Autodesk Inventor part; units mm, degrees
ref_plane "YZ Plane" through (0, 0, 0) normal (1, 0, 0) x (0, 1, 0)
ref_plane "XZ Plane" through (0, 0, 0) normal (0, 1, 0) x (-1, 0, 0)
ref_plane "XY Plane" through (0, 0, 0) normal (0, 0, 1) x (1, 0, 0)
sketch "Sketch1" plane through (0, 0, 0) normal (0, 0, 1) x (1, 0, 0)
  circle A0 centre (0, 0) radius 6.858
  dimension "d0" = 13.716
extrude "Extrusion1" add sketch "Sketch1" along normal blind 13.716
hole "Hole1" at (0, 0, 13.716) direction (0, 0, -1) diameter 12.192 depth 3.048
hole "Hole2" at (0, 0, 10.668) direction (0, 0, -1) diameter 11.43 depth 9.144
sketch "Sketch2" plane through (0, 0, 0) normal (1, 0, 0) x (0, 1, 0)
  line L0 (0, 0) -> (0, 6.35)
  circle A0 centre (0, 6.35) radius 1.7399
  dimension "d21" = 6.35
  dimension "d22" = 3.4798
extrude "Extrusion2" cut sketch "Sketch2" along normal through all both and the other way through all
sketch "Sketch3" plane through (0, 0, 0) normal (0, 0, -1) x (-1, 0, 0)
  line L0 (0, 0) -> (4.8942, 4.8942)
  line L1 (0, 0) -> (0, 6.9215) construction
sketch "Sketch4" plane through (0, 0, 0) normal (0, 1, 0) x (-1, 0, 0)
  point P0 (0, 0)
ref_plane "Work Plane1" through (-4.8942, 4.8942, 0) normal (-0.7071, 0.7071, 0) x (-0.7071, -0.7071, 0)
sketch "Sketch5" plane through (-4.8942, 4.8942, 0) normal (-0.7071, 0.7071, 0) x (-0.7071, -0.7071, 0)
  line L0 (0, 0) -> (0, 5.08)
  circle A0 centre (0, 5.08) radius 2.54
  dimension "d25" = 5.08
  dimension "d26" = 5.08
extrude "Extrusion3" cut sketch "Sketch5" against normal up to next
properties part number "Piston"
Source: CAD feature listing. Evaluate the final solid. Frame: model axes, mm. A direction names the side the tool comes from. Give positions to 0.01 mm unless a question says otherwise; leave off trailing zeros. Loops run counter-clockwise (first coordinate to the right, second up) from the corner with the lowest first, then second, coordinate; pieces in that order, holes last. Notation, with made-up numbers: (14, -39) - (51, -39) arc R12 ccw to (51, -28) - close; hole circle Ø7 at (73.5, 47). An arc over 180 degrees is marked (long way). Use CSV: the item, a comma, the result in double quotes. Start each with the question number.
1. Reachability of faces 1 (the cylindrical face through (5.07, -2.64, 6.03)), 2 (the cylindrical face through (6.54, -2.06, 6.76)) from +Z, -Z, +X, -X, +Y, -Y: full face, straight path, thin tool, end or side. Return the list, or none.
2. Ray query, L1, parallel to X at y = 0, z = 4.25 (3 decimals); L2, parallel to X at y = 0, z = 12.7; L3, parallel to Z at x = 4.75, y = 1. Return the intervals inside material, ascending.
3. Section A-A (z = 6.35). Output: boundary loops of the cut face in (x, y) (3 decimals), then the cut area to 3 significant figures.
4. Section C-C (y = -5). Output: boundary loops of the cut face in (x, z).
5. Section D-D (z = 2.25). Output: boundary loops of the cut face in (x, y) (3 decimals), then the cut area to 3 significant figures.
6. Pin query (flat end, axial travel): pin 1 (3 mm diameter, centred on x = 1.5, y = 5.5, fed in from +Z); pin 2 (5 mm diameter, centred on x = 3.5, z = 12, fed in from +Y); pin 3 (1.5 mm diameter, centred on x = 4.5, y = -0.5, fed in from +Z); pin 4 (1.5 mm diameter, centred on x = -2, z = 9.5, fed in from +Y). Return the tip coordinate at first contact, or that it passes through.
7. Section B-B (x = 0). Output: boundary loops of the cut face in (y, z) (3 decimals), then the cut area to 3 significant figures.
8. Draft query along Z for faces 3 (the cylindrical face through (-5.96, 2.53, 5.84)), 4 (the cylindrical face through (6.14, 1.66, 5.83)), 5 (the cylindrical face through (-6.044, 0.794, 12.171)), 6 (the flat face through (-5, -4, 13.716)). Return one class per face: +Z half, -Z half, draft (parallel to the pull), parting line (faces both ways), or undercut.
Response:
1,face 1,"+Z"
1,face 2,"+Z, -Z"
2,L1,"-6.858 to -5.715, 5.715 to 6.858"
2,L2,"-6.86 to -6.1, 6.1 to 6.86"
2,L3,"0 to 1.52"
3,outline,"(-6.634, -1.74) arc R6.858 ccw to (6.634, -1.74) - (5.444, -1.74) arc R5.715 cw to (-5.444, -1.74) - close; (-6.634, 1.74) - (-5.444, 1.74) arc R5.715 cw to (-5.285, 2.174) - (-6.149, 3.038) arc R6.858 ccw to start; (-3.038, 6.149) - (-2.174, 5.285) arc R5.715 cw to (5.444, 1.74) - (6.634, 1.74) arc R6.858 ccw to start"
3,area,"31.9 mm²"
4,outline,"(-4.69, 0) - (4.69, 0) - (4.69, 13.72) - (3.49, 13.72) - (3.49, 10.67) - (2.77, 10.67) - (2.77, 1.52) - (-2.77, 1.52) - (-2.77, 10.67) - (-3.49, 10.67) - (-3.49, 13.72) - (-4.69, 13.72) - close"
5,outline,"circle Ø13.716 at (0, 0); hole circle Ø11.43 at (0, 0)"
5,area,"45.1 mm²"
6,pin 1,"z = 13.72"
6,pin 2,"y = 6.78"
6,pin 3,"z = 1.52"
6,pin 4,"y = 6.74"
7,outline,"(-6.858, 0) - (6.858, 0) - (6.858, 13.716) - (6.096, 13.716) - (6.096, 10.668) - (5.715, 10.668) - (5.715, 1.524) - (-5.715, 1.524) - (-5.715, 10.668) - (-6.096, 10.668) - (-6.096, 13.716) - (-6.858, 13.716) - close"
7,area,"46.5 mm²"
8,face 3,"undercut"
8,face 4,"undercut"
8,face 5,"draft"
8,face 6,"+Z half"
